Read the model definition and answer for the solid it produces. Units are mm, in the model's axes. Face numbers are marked on the shaded views. A direction names the side the tool comes from. Coordinates: 2 decimals unless noted, no trailing zeros. Write each loop counter-clockwise with the first axis right and the second up, starting at its lowest first coordinate (ties: lowest second). Pieces come first, ordered by that corner, then holes.
1) Find the intervals of material crossed by line 1 (X direction, y = 15.5, z = 90.65); line 2 (Z direction, x = -93.7, y = 15.5); line 3 (Y direction, x = -12, z = 19), in increasing order.
2) The part is cut by section D-D (x = -72). Determine the outline of the cut face in (y, z).
3) Each of these flat-tipped pins is pushed along its axis until it touches: pin 1 Ø15 at (x, y) = (-7.5, 17.5) entering from -Z; pin 2 Ø15 at (y, z) = (16, 5) entering from +X; pin 3 Ø4 at (x, y) = (-10, 15.5) entering from +Z; pin 4 Ø12 at (y, z) = (3, 73.5) entering from -X. Where does it stop, or does it pass through?
4) The part is cut by section C-C (z = 58.5). Determine the outline of the cut face in (x, y).
5) Which of the six approach directions +Z, -Z, +X, -X, +Y, -Y give full straight-line access (tool end or side, diameter ignored) to the marked faces 1, 2, 3 and 4?
6) The part is cut by section A-A (y = 12). Determine the outline of the cut face in (x, z), then the cut area to 3 significant figures.
7) The part is cut by section B-B (x = -10). Determine the outline of the cut face in (y, z).
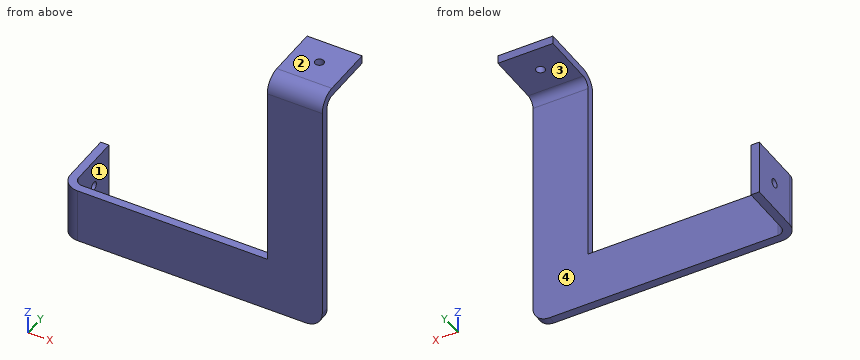
Autodesk Inventor part; units mm, degrees
ref_plane "YZ Plane" through (0, 0, 0) normal (1, 0, 0) x (0, 1, 0)
ref_plane "XZ Plane" through (0, 0, 0) normal (0, 1, 0) x (-1, 0, 0)
ref_plane "XY Plane" through (0, 0, 0) normal (0, 0, 1) x (1, 0, 0)
sketch "草圖1" plane through (0, 0, 0) normal (0, 1, 0) x (-1, 0, 0)
  line L0 (0, 0) -> (0, 92.5)
  line L1 (0, 92.5) -> (20, 92.5)
  line L2 (20, 92.5) -> (20, 20)
  line L3 (20, 20) -> (95, 20)
  line L4 (95, 20) -> (95, 0)
  line L5 (95, 0) -> (0, 0)
  dimension "d0" = 92.5
  dimension "d1" = 95
  dimension "d2" = 20
  dimension "d3" = 20
extrude "平板1" add sketch "草圖1" along normal blind 3
fillet "轉角外圓角1" radius 6 1 edges at (0, 1.5, 0)
sketch "草圖2" plane through (0, 0, 89.5) normal (0, 0, 1) x (1, 0, 0)
  line L0 (-20, 0) -> (0, 0)
  line L1 (0, 0) -> (0, 25)
  line L2 (0, 25) -> (-20, 25)
  line L3 (-20, 25) -> (-20, 0)
edge flange "凸緣1" height 25 angle 90 thickness 3 bend radius 3 thickness toward (0, 0, 1) relief tear relief width 3 relief depth 1.5 corner gap 3 corner form 0 edges at (-10, 3, 92.5) (-95, 3, 10) wall of the first edge with corners at (-20, 0, 89.5) (0, 0, 89.5) (0, 25, 89.5) (-20, 25, 89.5)
bend "折彎1"
corner "轉角1"
sketch "草圖3" plane through (-92, 25, 20) normal (1, 0, 0) x (0, 0, -1)
  line L0 (20, 0) -> (0, 0)
  line L1 (20, -19) -> (20, 0)
  point P0 (20, -25)
  point P1 (10, -9.5)
  point P2 (10, 0)
  point P3 (20, -9.5)
hole "孔1" at (-92, 15.5, 10) direction (-1, 0, 0) diameter 3.2 end through all
sketch "草圖4" plane through (0, 25, 89.5) normal (0, 0, -1) x (-1, 0, 0)
  line L0 (20, 0) -> (0, 0)
  line L1 (20, -19) -> (20, 0)
  point P0 (0, -25)
  point P1 (10, -9.5)
  point P2 (10, 0)
  point P3 (20, -9.5)
hole "孔2" at (-10, 15.5, 89.5) direction (0, 0, 1) diameter 3.2 end through all
equation "\"d21\" = 厚度"
equation "\"d28\" = 厚度"
equation "\"d4\" = 厚度"
equation "\"d6\" = 折彎離隙寬度"
equation "\"d7\" = 折彎離隙深度"
equation "\"d8\" = 最小剩餘"
equation "\"d9\" = 轉移半徑"
equation "\"d12\" = 折彎半徑"
equation "\"d13\" = 轉角離隙大小"
equation "\"d14\" = 間隙大小"
equation "\"d15\" = Jacobi半徑大小"
equation "\"折彎半徑\" = 厚度"
equation "\"折彎離隙寬度\" = 厚度"
equation "\"折彎離隙深度\" = 0.5 * 厚度"
equation "\"轉角離隙大小\" = 4 * 厚度"
equation "\"最小剩餘\" = 2 * 厚度"
equation "\"轉移半徑\" = 折彎半徑"
equation "\"Jacobi半徑大小\" = 折彎半徑"
equation "\"間隙大小\" = 厚度"
properties part number "鋁擠加強肋"
Reported:
1. line 1: x = -20 to -11.6, -8.4 to 0
1. line 2: z = 0 to 8.4, 11.6 to 20
1. line 3: y = 0 to 3
2. outline: (0, 0) - (3, 0) - (3, 20) - (0, 20) - close
3. pin 1: stops at z = 89.5
3. pin 2: stops at x = -92
3. pin 3: stops at z = 92.5
3. pin 4: stops at x = -20
4. outline: (-20, 0) - (0, 0) - (0, 3) - (-20, 3) - close
5. face 1: +Z, -Z, +X, +Y
5. face 2: +Z, +X, -X, +Y, -Y
5. face 3: -Z, +X, -X, +Y
5. face 4: -Z, +X, +Y
6. outline: (-95, 0) - (-92, 0) - (-92, 20) - (-95, 20) - close; (-20, 89.5) - (0, 89.5) - (0, 92.5) - (-20, 92.5) - close
6. area: 120 mm2
7. outline: (0, 0) - (3, 0) - (3, 86.5) arc R3 cw to (6, 89.5) - (13.9, 89.5) - (13.9, 92.5) - (6, 92.5) arc R6 ccw to (0, 86.5) - close; (17.1, 89.5) - (25, 89.5) - (25, 92.5) - (17.1, 92.5) - close
